```python
from build123d import *

# Parameters (mm, degrees)
SKETCH1_W           = 37
SKETCH1_H           = 18.6
BOSS_EXTRUDE1_DEPTH = 22.44
SKETCH6_W           = 5
SKETCH6_H           = 2.8
BOSS_EXTRUDE2_DEPTH = 4.8
CUT_EXTRUDE1_REACH  = 36.072
SKETCH7_R           = 1.5
SKETCH8_R           = 2.7
BOSS_EXTRUDE3_DEPTH = 9


with BuildPart() as part:
    # Sketch1 → Boss-Extrude1 (new body)
    with BuildSketch(Plane.XY):
        Rectangle(SKETCH1_W, SKETCH1_H)
    extrude(amount=BOSS_EXTRUDE1_DEPTH)

    # Sketch6 → Boss-Extrude2 (add)
    with BuildSketch(Plane(origin=(18.5, 0, 0), x_dir=(0, 0, -1), z_dir=(1, 0, 0))):
        with Locations((-11.22, 0)):
            Rectangle(SKETCH6_W, SKETCH6_H)
    extrude(amount=BOSS_EXTRUDE2_DEPTH)

    # Sketch7 → Cut-Extrude1 (cut, up to next)
    with BuildSketch(Plane(origin=(0, 1.4, 0), x_dir=(1, 0, 0), z_dir=(0, 1, 0)), mode=Mode.PRIVATE) as cut_extrude1_sk1:
        with Locations(Location((20.9, -11.22, 0), (0, 0, 270))):
            Circle(SKETCH7_R)
    cut_extrude1_tool1 = extrude(cut_extrude1_sk1.sketch, amount=-CUT_EXTRUDE1_REACH, mode=Mode.PRIVATE) & part.part
    add(cut_extrude1_tool1.solids().sort_by_distance((20.9, 1.4, 11.22))[0], mode=Mode.SUBTRACT)

    # Sketch8 → Boss-Extrude3 (add)
    with BuildSketch(Plane(origin=(0, 9.3, 0), x_dir=(1, 0, 0), z_dir=(0, 1, 0))):
        with Locations((6.9, -11.22)):
            Circle(SKETCH8_R)
    boss_extrude3 = extrude(amount=BOSS_EXTRUDE3_DEPTH)

    # Mirror1: Boss-Extrude3 across plane
    add(boss_extrude3.mirror(Plane.ZX))


solid = part.part
```
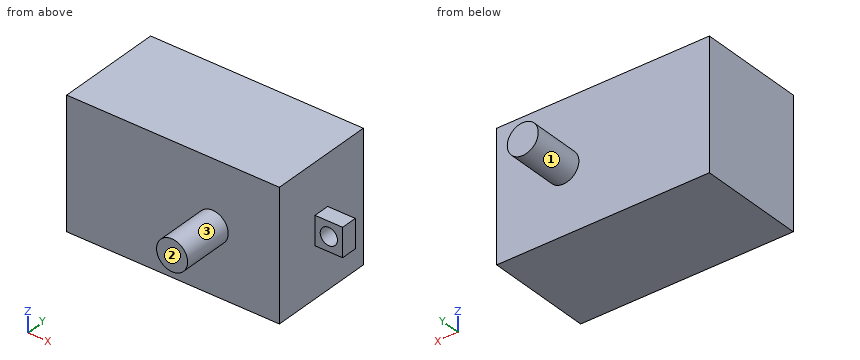
Geometry check sheet. Reference: the model listing, model coordinates, mm. Face numbers are marked on the shaded views. A direction names the side the tool comes from. Coordinates: 2 decimals unless noted, no trailing zeros. Write each loop counter-clockwise with the first axis right and the second up, starting at its lowest first coordinate (ties: lowest second). Pieces come first, ordered by that corner, then holes. Notation, with made-up numbers: M 32.5,32 L 39.5,32 A24 cw 39.5,54 Z; hole C -38.5,14 d11. An arc over 180 degrees is marked long. Answer as a JSON object with one key per item and string values.
1. Scan lines: L1, parallel to X at y = 0.05, z = 11.22; L2, parallel to Y at x = 12, z = 12.5; L3, parallel to X at y = -8, z = 10.75. Record each from-to range of solid material in increasing order.
Answers below:
{"L1": "x = -18.5 to 19.4, 22.4 to 23.3", "L2": "y = -9.3 to 9.3", "L3": "x = -18.5 to 18.5"}
2. Section check A-A, the plane z = 11.22. Enter the section's corners in (x, y), plus the area to 3 significant figures.
Answers below:
{"outline": "M -18.5,-9.3 L 4.2,-9.3 L 4.2,-18.3 L 9.6,-18.3 L 9.6,-9.3 L 18.5,-9.3 L 18.5,-1.4 L 19.4,-1.4 L 19.4,1.4 L 18.5,1.4 L 18.5,9.3 L 9.6,9.3 L 9.6,18.3 L 4.2,18.3 L 4.2,9.3 L -18.5,9.3 Z; M 22.4,-1.4 L 23.3,-1.4 L 23.3,1.4 L 22.4,1.4 Z", "area": "790 mm²"}
3. Tool access check on the marked faces 1, 2 and 3. Record the directions out of +Z, -Z, +X, -X, +Y, -Y that give a thin tool (end or side, any length) a straight path to the whole face; none if there is none.
Answers below:
{"face 1": "+Y", "face 2": "+Z, -Z, +X, -X, -Y", "face 3": "-Y"}
4. Section check D-D, the plane y = 14.5. Enter the section's corners in (x, z), plus the area to 3 significant figures.
Answers below:
{"outline": "C 6.9,11.22 d5.4", "area": "22.9 mm²"}
5. Section check C-C, the plane x = 6.9. Enter the section's corners in (y, z), plus the area to 3 significant figures.
Answers below:
{"outline": "M -18.3,8.52 L -9.3,8.52 L -9.3,0 L 9.3,0 L 9.3,8.52 L 18.3,8.52 L 18.3,13.92 L 9.3,13.92 L 9.3,22.44 L -9.3,22.44 L -9.3,13.92 L -18.3,13.92 Z", "area": "515 mm²"}
6. Go/stop test with flat-tipped pins: pin 1 Ø6.5 at (x, z) = (2.5, 6.5) entering from -Y; pin 2 Ø5.5 at (x, z) = (21, 10.5) entering from +Y; pin 3 Ø0.8 at (x, y) = (21.5, 0) entering from -Z. Record where each tip stops, or that it passes through.
Answers below:
{"pin 1": "stops at y = -9.3", "pin 2": "stops at y = 9.3", "pin 3": "stops at z = 8.72"}
7. Section check B-B, the plane x = 20.9. Enter the section's corners in (y, z), plus the area to 3 significant figures.
Answers below:
{"outline": "M -1.4,8.72 L 1.4,8.72 L 1.4,9.72 L -1.4,9.72 Z; M -1.4,12.72 L 1.4,12.72 L 1.4,13.72 L -1.4,13.72 Z", "area": "5.60 mm²"}
